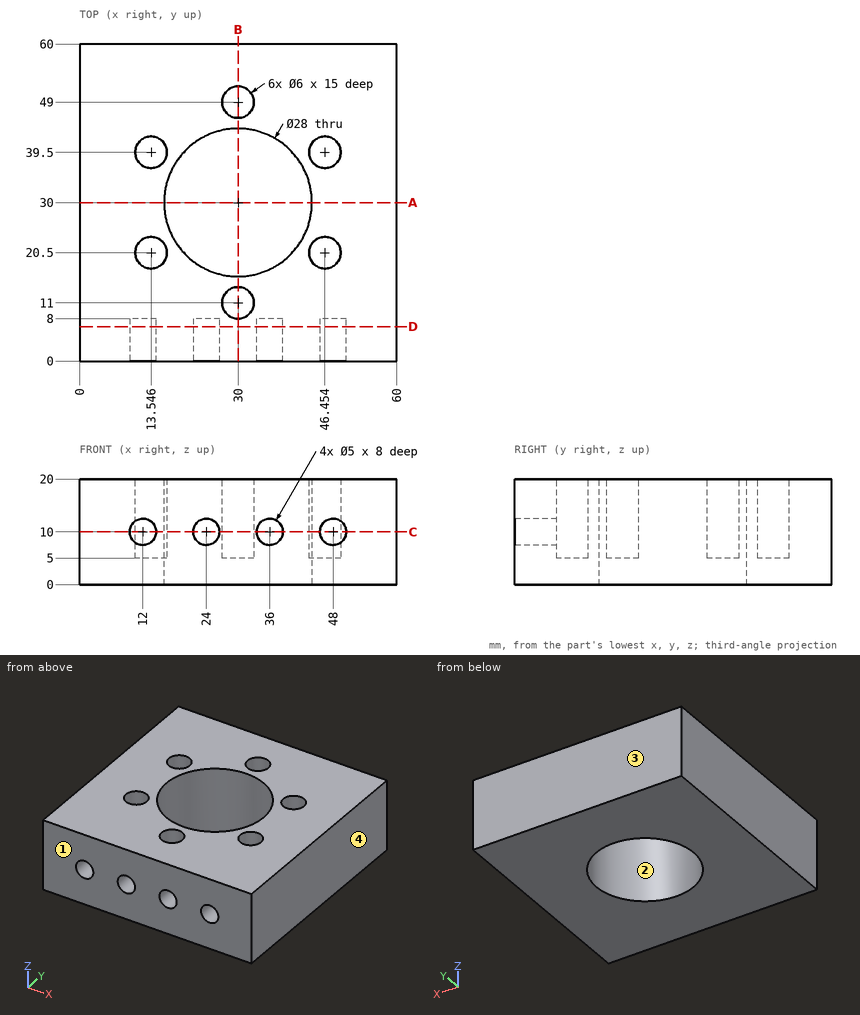
The figure shows three views and two pictorial views of one solid part (mm, origin at its lowest corner). Answer the questions. Round coordinates to 2 decimals unless told otherwise and drop trailing zeros. Order: outer loops, then holes, each group sorted by start corner. A loop starts at its lowest first (then second) coordinate and runs counter-clockwise, first axis right, second up. Notation, with made-up numbers: M 21.25,73 L 50.25,73 A13 ccw 50.25,98 Z; hole C -1,1.5 d11. An arc over 180 degrees is marked long. Put each result on its own line as item: value. Start each with the question number.
Q1. For a pull along Y with two mould halves and no side action, classify the marked faces 1, 2, 3 and 4 as pulls with the +Y half, pulls with the -Y half, needs draft (parallel to the pull), parting line crosses it, or undercut.
Q2. Flat-ended cylindrical pins translate along their axes: pin 1 (6.5 mm diameter, centred on x = 47.5, y = 38.5, fed in from +Z); pin 2 (1.8 mm diameter, centred on x = 31, y = 11, fed in from +Z); pin 3 (22.5 mm diameter, centred on x = 30, y = 30, fed in from +Z); pin 4 (2.5 mm diameter, centred on x = 23.5, z = 9, fed in from -Y). Find the tip coordinate at first contact, or state that the pin passes through.
Q3. Section A-A, the plane y = 30 is taken. Write down the section's boundary in (x, z), and give its area (3 significant figures).
Q4. Section B-B, the plane x = 30 is taken. Write down the section's boundary in (y, z), and give its area (3 significant figures).
Q5. Straight lines are drawn through the part: L1, parallel to X at y = 4.25, z = 10; L2, parallel to Y at x = 30, z = 12.5; L3, parallel to Y at x = 46.5, z = 14.25. For each, find the intervals that lie inside material, in ascending order. Write a range as [from, to].
Q6. Section C-C, the plane z = 10 is taken. Write down the section's boundary in (x, y) (1 decimal).
Q7. Section D-D, the plane y = 6.5 is taken. Write down the section's boundary in (x, z).
Findings below:
1. face 1: pulls with the -Y half
1. face 2: undercut
1. face 3: pulls with the +Y half
1. face 4: needs draft
2. pin 1: stops at z = 20
2. pin 2: stops at z = 5
2. pin 3: passes through
2. pin 4: stops at y = 8
3. outline: M 0,0 L 16,0 L 16,20 L 0,20 Z; M 44,0 L 60,0 L 60,20 L 44,20 Z
3. area: 640 mm^2
4. outline: M 0,0 L 16,0 L 16,20 L 14,20 L 14,5 L 8,5 L 8,20 L 0,20 Z; M 44,0 L 60,0 L 60,20 L 52,20 L 52,5 L 46,5 L 46,20 L 44,20 Z
4. area: 460 mm^2
5. L1: x = [0, 9.5], [14.5, 21.5], [26.5, 33.5], [38.5, 45.5], [50.5, 60]
5. L2: y = [0, 8], [14, 16], [44, 46], [52, 60]
5. L3: y = [0, 17.5], [23.5, 36.5], [42.5, 60]
6. outline: M 0,0 L 9.5,0 L 9.5,8 L 14.5,8 L 14.5,0 L 21.5,0 L 21.5,8 L 26.5,8 L 26.5,0 L 33.5,0 L 33.5,8 L 38.5,8 L 38.5,0 L 45.5,0 L 45.5,8 L 50.5,8 L 50.5,0 L 60,0 L 60,60 L 0,60 Z; hole C 13.5,20.5 d6; hole C 13.5,39.5 d6; hole C 30,30 d28; hole C 30,11 d6; hole C 30,49 d6; hole C 46.5,20.5 d6; hole C 46.5,39.5 d6
7. outline: M 0,0 L 60,0 L 60,20 L 0,20 Z; hole C 12,10 d5; hole C 24,10 d5; hole C 36,10 d5; hole C 48,10 d5
